Check sheet for the drawn part. Datum: minimum x, y, z corner. Units: mm. A direction names the side the tool comes from. Give positions to 0.01 mm unless a question says otherwise; leave off trailing zeros. Loops run counter-clockwise (first coordinate to the right, second up) from the corner with the lowest first, then second, coordinate; pieces in that order, holes last. Notation, with made-up numbers: (6.5, 52) - (42.5, 52) arc R23 ccw to (42.5, 85) - close; hole circle Ø1 at (5.25, 65). An arc over 180 degrees is marked (long way). Answer in a Markdown table with one row per item.
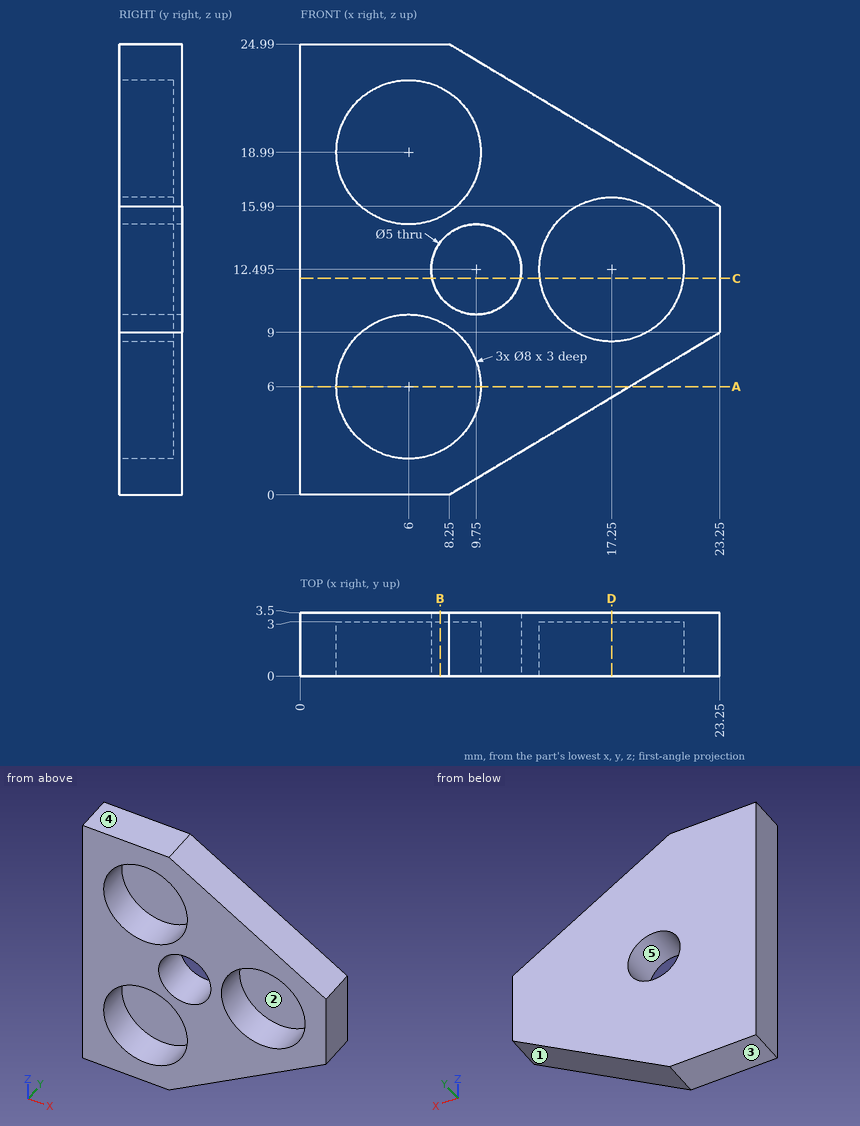
Q1. Thickness scan on line 1 (Z direction, x = 6, y = 2.45); line 2 (Z direction, x = 7.75, y = 0.75) (1 decimal); line 3 (X direction, y = 2.7, z = 10.75). Record the ranges inside material, lowest first.
Completed:
| item | result |
|---|---|
| line 1 | 0 to 2, 10 to 14.99, 22.99 to 24.99 |
| line 2 | 0 to 2.4, 9.6 to 11, 14 to 15.4, 22.6 to 25 |
| line 3 | 0 to 7.96, 11.54 to 13.65, 20.85 to 23.25 |
Q2. Sectioned sample at A-A (z = 6). Record the cut outline in (x, y).
Completed:
| item | result |
|---|---|
| outline | (0, 0) - (2, 0) - (2, 3) - (10, 3) - (10, 0) - (18.25, 0) - (18.25, 3.5) - (0, 3.5) - close |
Q3. Sectioned sample at B-B (x = 7.75). Record the cut outline in (y, z) (1 decimal).
Completed:
| item | result |
|---|---|
| outline | (0, 0) - (3.5, 0) - (3.5, 11) - (0, 11) - (0, 9.6) - (3, 9.6) - (3, 2.4) - (0, 2.4) - close; (0, 14) - (3.5, 14) - (3.5, 25) - (0, 25) - (0, 22.6) - (3, 22.6) - (3, 15.4) - (0, 15.4) - close |
Q4. Tool access check on the marked faces 1 and 2. Record the directions out of +Z, -Z, +X, -X, +Y, -Y that give a thin tool (end or side, any length) a straight path to the whole face; none if there is none.
Completed:
| item | result |
|---|---|
| face 1 | -Z, +X, +Y, -Y |
| face 2 | -Y |
Q5. Sectioned sample at D-D (x = 17.25). Record the cut outline in (y, z) (1 decimal).
Completed:
| item | result |
|---|---|
| outline | (0, 5.4) - (3.5, 5.4) - (3.5, 19.6) - (0, 19.6) - (0, 16.5) - (3, 16.5) - (3, 8.5) - (0, 8.5) - close |
Q6. Go/stop test with flat-tipped pins: P1, Ø4, axis at x = 9.75, z = 12.5, coming from the -Y side; P2, Ø6.5, axis at x = 17.5, z = 14, coming from the -Y side; P3, Ø2, axis at x = 15, y = 2, coming from the -Z side; P4, Ø6.5, axis at x = 6, z = 6, coming from the -Y side. Record where each tip stops, or that it passes through.
Completed:
| item | result |
|---|---|
| P1 | through |
| P2 | y = 0 |
| P3 | z = 3.45 |
| P4 | y = 3 |
Q7. Draft check along Z on the marked faces 3, 4 and 5. Enter one of: +Z half, -Z half, draft (parallel to the pull), parting line (faces both ways), or undercut.
Completed:
| item | result |
|---|---|
| face 3 | -Z half |
| face 4 | +Z half |
| face 5 | undercut |
Q8. Sectioned sample at C-C (z = 12). Record the cut outline in (x, y).
Completed:
| item | result |
|---|---|
| outline | (0, 0) - (7.3, 0) - (7.3, 3.5) - (0, 3.5) - close; (12.2, 0) - (13.28, 0) - (13.28, 3) - (21.22, 3) - (21.22, 0) - (23.25, 0) - (23.25, 3.5) - (12.2, 3.5) - close |
